```python
from build123d import *
from build123d.topology import SkipClean

# Parameters (mm, degrees)
SKETCH1_W               = 700
SKETCH1_H               = 400
BOSS_EXTRUDE2_DEPTH     = 50
BOSS_EXTRUDE3_DEPTH     = 10
CUT_EXTRUDE1_DEPTH      = 788.223691227
CUT_EXTRUDE1_DEPTH_BACK = 788.223691227
LPATTERN1_COUNT         = 6
LPATTERN1_PITCH         = 100


with BuildPart() as part:
    # Sketch1 → Boss-Extrude2 (new body)
    with BuildSketch(Plane.XY):
        with Locations((350, 200)):
            Rectangle(SKETCH1_W, SKETCH1_H)
    extrude(amount=BOSS_EXTRUDE2_DEPTH)

    # Sketch2 → Boss-Extrude3 (add)
    with BuildSketch(Plane(origin=(650, 0, 0), x_dir=(0, 0, -1), z_dir=(1, 0, 0))):
        with BuildLine():
            Line((-50, 0), (-192.927810409, 0))
            Line((-192.927810409, 0), (-192.927810409, 12.5))
            ThreePointArc((-192.927810409, 12.5), (-5.427810409, 200), (-192.927810409, 387.5))
            Line((-192.927810409, 387.5), (-192.927810409, 400))
            Line((-192.927810409, 400), (-50, 400))
            Line((-50, 400), (0, 400))
            Line((0, 400), (0, 0))
            Line((0, 0), (-50, 0))
        make_face()
    boss_extrude3 = extrude(amount=BOSS_EXTRUDE3_DEPTH)

    # Sketch3 → Cut-Extrude1 (cut, two sides: drawn at the far end of the back side and taken through both)
    with SkipClean():  # the faces are left unmerged after this step: merging them gives an invalid solid
        with BuildSketch(Plane(origin=(650, 0, 0), x_dir=(0, 0, -1), z_dir=(1, 0, 0)).offset(-CUT_EXTRUDE1_DEPTH_BACK)):
            with BuildLine():
                Line((-50, 78.641477383), (-50, 321.358522617))
                ThreePointArc((-50, 321.358522617), (-5.427810409, 200), (-50, 78.641477383))
            make_face()
        extrude(amount=CUT_EXTRUDE1_DEPTH + CUT_EXTRUDE1_DEPTH_BACK, mode=Mode.SUBTRACT)

    # LPattern1: Boss-Extrude3 ×6
    with Locations(*[(-i * LPATTERN1_PITCH, 0, 0) for i in range(1, LPATTERN1_COUNT)]):
        add(boss_extrude3)


solid = part.part
```
Geometry check sheet. Reference: the model listing, model coordinates, mm. A direction names the side the tool comes from. Coordinates: 2 decimals unless noted, no trailing zeros. Loops run counter-clockwise (first coordinate to the right, second up) from the corner with the lowest first, then second, coordinate; pieces in that order, holes last.
Item 1: Sectioned sample at D-D, the plane z = 99. Count the separate pieces of the cut face and the enclosed holes in it, then the cut area to 3 significant figures.
Item 2: Thickness scan on line 1 (X direction, y = 378.5, z = 93); line 2 (Z direction, x = 472, y = 360); line 3 (Y direction, x = 158.5, z = 175.5). Record the ranges inside material, lowest first.
Item 3: Go/stop test with flat-tipped pins: pin 1 Ø23.5 at (y, z) = (27.5, 138.5) entering from -X; pin 2 Ø8 at (x, y) = (75.5, 57.5) entering from +Z. Record where each tip stops, or that it passes through.
Item 4: Access from +Z, -Z, +X, -X, +Y, -Y to the whole of each face (thin tool, end or side, straight path). Record for faces 4 (the face through (400, 400, 46)), 5 (the face through (160, 22, 105)), 6 (the face through (74, 40, 50)).
Item 5: Sectioned sample at A-A, the plane z = 16. Record the boundary of the cut face in (x, y), then the cut area to 3 significant figures.
Item 6: Sectioned sample at C-C, the plane y = 70. Record the boundary of the cut face in (x, z).
Item 7: Release check for a two-part mould opening along X. For faces 1 (the face through (560, 22, 105)), 2 (the face through (0, 197, 2)), 3 (the face through (400, 0, 32)) record: released by +X, released by -X, zero draft, split by the parting line, or undercut.
Item 8: Sectioned sample at B-B, the plane x = 519. Record the boundary of the cut face in (y, z), then the cut area to 3 significant figures.
Check result:
1. separate pieces: 12
1. enclosed holes: 0
1. area: 4,530 mm2
2. line 1: x = 150 to 160, 250 to 260, 350 to 360, 450 to 460, 550 to 560, 650 to 660
2. line 2: z = 0 to 50
2. line 3: y = 0 to 13.31, 386.69 to 400
3. pin 1: stops at x = 150
3. pin 2: stops at z = 50
4. face 4: +Z, -Z, +X, -X, +Y
4. face 5: +Z, +Y, -Y
4. face 6: +Z, -X, +Y, -Y
5. outline: (0, 0) - (700, 0) - (700, 137.93) - (0, 137.93) - close; (0, 262.07) - (700, 262.07) - (700, 400) - (0, 400) - close
5. area: 193,000 mm2
6. outline: (0, 0) - (700, 0) - (700, 50) - (660, 50) - (660, 57.81) - (650, 57.81) - (650, 50) - (560, 50) - (560, 57.81) - (550, 57.81) - (550, 50) - (460, 50) - (460, 57.81) - (450, 57.81) - (450, 50) - (360, 50) - (360, 57.81) - (350, 57.81) - (350, 50) - (260, 50) - (260, 57.81) - (250, 57.81) - (250, 50) - (160, 50) - (160, 57.81) - (150, 57.81) - (150, 50) - (0, 50) - close
7. face 1: undercut
7. face 2: released by -X
7. face 3: zero draft
8. outline: (0, 0) - (400, 0) - (400, 50) - (321.36, 50) arc R187.5 cw to (78.64, 50) - (0, 50) - close
8. area: 12,600 mm2
